Design review of the part built by this model. Coordinates are the model's own, in mm. Face numbers are marked on the shaded views. A direction names the side the tool comes from. Give positions to 0.01 mm unless a question says otherwise; leave off trailing zeros. Loops run counter-clockwise (first coordinate to the right, second up) from the corner with the lowest first, then second, coordinate; pieces in that order, holes last. Notation, with made-up numbers: (-20.75, 75) -> (9.25, 75) arc R4 ccw to (9.25, 80) -> close; hole circle Ø7 at (21, 3.25). An arc over 180 degrees is marked (long way). Answer in a Markdown table with one row per item. Add a question column.
(1) Consider section A-A on z = 2. Count the separate pieces of the cut face and the enclosed holes in it, then the cut area to 3 significant figures.
(2) For pin 1 (6.5 mm diameter, centred on x = 49, y = -1.5, fed in from +Z); pin 2 (0.6 mm diameter, centred on x = -0.5, z = 6.5, fed in from -Y); pin 3 (5 mm diameter, centred on x = 33, y = 8.5, fed in from +Z), all flat-tipped, find the tip position at first contact; note any pin that passes through.
(3) For line 1 (Z direction, x = 23, y = 21.5); line 2 (X direction, y = 5, z = 6.25); line 3 (X direction, y = 2.5, z = 2.75), list the stretches that pass through material, from the lowest coordinate up.
(4) Consider section C-C on x = 23. Write out the cut boundary in (y, z), then the cut area to 3 significant figures.
(5) Consider section D-D on y = 26.5. Write out the cut boundary in (x, z), then the cut area to 3 significant figures.
(6) For the marked faces 1, 2 and 3, list the 3-axis set-ups (+Z, -Z, +X, -X, +Y, -Y) from which the entire face can be reached by the end or side of a thin tool; tool diameter is ignored.
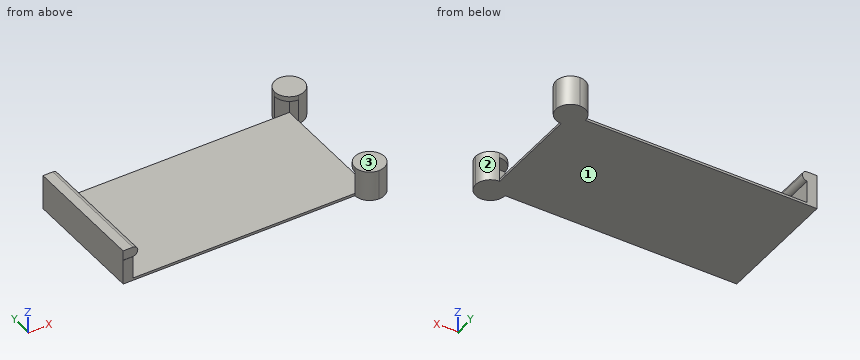
Autodesk Fusion 360 part; units mm, degrees
sketch "Sketch1" plane through (0, 0, 0) normal (0, 0, 1) x (1, 0, 0)
  line L0 (0, 0) -> (48.35, 0)
  line L1 (48.35, 0) -> (48.35, 25.75)
  line L2 (48.35, 25.75) -> (0, 25.75)
  line L3 (0, 25.75) -> (0, 0)
  line L4 (51.35, 22.75) -> (45.35, 22.75)
  line L5 (45.35, 22.75) -> (45.35, 28.75)
  line L6 (45.35, 28.75) -> (51.35, 28.75)
  line L7 (51.35, 28.75) -> (51.35, 22.75)
  line L8 (51.35, 22.75) -> (45.35, 28.75) construction
  line L9 (45.35, 22.75) -> (51.35, 28.75) construction
  line L10 (51.35, -3) -> (45.35, -3)
  line L11 (45.35, -3) -> (45.35, 3)
  line L12 (45.35, 3) -> (51.35, 3)
  line L13 (51.35, 3) -> (51.35, -3)
  line L14 (51.35, -3) -> (45.35, 3) construction
  line L15 (45.35, -3) -> (51.35, 3) construction
  line L16 (0, 0) -> (-2, 0)
  line L17 (-2, 0) -> (-2, 25.75)
  line L18 (-2, 25.75) -> (0, 25.75)
  line L19 (0, 25.75) -> (0, 0)
  point P0 (48.35, 25.75)
  point P1 (48.35, 0)
  dimension "d1" = 48.35
  dimension "d2" = 25.75
  dimension "d3" = 6
  dimension "d4" = 6
  dimension "d5" = 6
  dimension "d6" = 6
  dimension "d7" = 2
  dimension "d8" = 25.75
extrude "Extrude1" add sketch "Sketch1" along normal blind 0.5
extrude "Extrude2" add sketch "Sketch1" along normal blind 5.1 contours L3 L16 L17 L18 L19
sketch "Sketch2" plane through (0, 0, 5.1) normal (0, 0, 1) x (1, 0, 0)
  line L0 (0, 25.75) -> (-2, 25.75)
  line L1 (-2, 25.75) -> (-2, 0)
  line L2 (-2, 0) -> (0, 0)
  line L3 (0, 0) -> (0, 25.75)
  line L4 (-2, 25.75) -> (1, 25.75)
  line L5 (1, 25.75) -> (1, 0.05)
  line L6 (1, 0.05) -> (-2, 0.05)
  line L7 (-2, 0.05) -> (-2, 25.75)
  dimension "d13" = 3
  dimension "d14" = 25.7
extrude "Extrude3" add sketch "Sketch2" along normal blind 2 contours L0 L1 L3 L4 L6 L7 | L3 L4 L5 L6
fillet "Fillet1" radius 1 2 edges at (1, 12.9, 7.1) (1, 12.9, 5.1)
extrude "Extrude4" add sketch "Sketch1" along normal blind 5.1 contours L0 L1 L10 L11 L12 L13 | L1 L2 L4 L5 L6 L7
sketch "Sketch3" plane through (0, 0, 5.1) normal (0, 0, 1) x (1, 0, 0)
  line L0 (51.35, 3) -> (48.35, 3)
  line L1 (48.35, 3) -> (48.35, 0)
  line L2 (48.35, 0) -> (45.35, 0)
  line L3 (45.35, 0) -> (45.35, -3)
  line L4 (45.35, -3) -> (51.35, -3)
  line L5 (51.35, -3) -> (51.35, 3)
  line L6 (51.35, -3) -> (45.35, -3)
  line L7 (45.35, -3) -> (45.35, 3)
  line L8 (45.35, 3) -> (51.35, 3)
  line L9 (51.35, 3) -> (51.35, -3)
  line L10 (51.35, 28.75) -> (45.35, 28.75)
  line L11 (45.35, 28.75) -> (45.35, 22.75)
  line L12 (45.35, 22.75) -> (51.35, 22.75)
  line L13 (51.35, 22.75) -> (51.35, 28.75)
  point P0 (51.35, 28.75)
  dimension "d21" = 6
  dimension "d22" = 6
  dimension "d23" = 6
  dimension "d24" = 6
extrude "Extrude5" add sketch "Sketch3" along normal blind 1
fillet "Fillet2" radius 3 6 edges at (51.35, -3, 3.05) (51.35, 3, 3.05) (45.35, -3, 3.05) (51.35, 22.75, 3.05) (45.35, 28.75, 3.05) (51.35, 28.75, 3.05)
fillet "Fillet3" radius 3 2 edges at (45.35, 22.75, 5.6) (45.35, 3, 5.6)
Values follow:
| question | item | result |
|---|---|---|
| 1 | separate pieces | 3 |
| 1 | enclosed holes | 0 |
| 1 | area | 93.9 mm2 |
| 2 | pin 1 | z = 6.1 |
| 2 | pin 2 | y = 0.05 |
| 2 | pin 3 | z = 0.5 |
| 3 | line 1 | 0 to 0.5 |
| 3 | line 2 | -2 to 0.99 |
| 3 | line 3 | -2 to 0, 48.35 to 50.01 |
| 4 | outline | (0, 0) -> (25.75, 0) -> (25.75, 0.5) -> (0, 0.5) -> close |
| 4 | area | 12.9 mm2 |
| 5 | outline | (45.45, 0) -> (51.25, 0) -> (51.25, 6.1) -> (45.45, 6.1) -> close |
| 5 | area | 35.4 mm2 |
| 6 | face 1 | -Z, +X, -X, +Y, -Y |
| 6 | face 2 | +Z, -Z, +X |
| 6 | face 3 | +Z, +X, +Y, -Y |
